Read the model definition and answer for the solid it produces. Units are mm, in the model's axes. Face numbers are marked on the shaded views. A direction names the side the tool comes from. Give positions to 0.01 mm unless a question says otherwise; leave off trailing zeros. Write each loop counter-clockwise with the first axis right and the second up, starting at its lowest first coordinate (ties: lowest second). Pieces come first, ordered by that corner, then holes. Notation, with made-up numbers: (-37.5, -18.5) - (19.5, -18.5) arc R21 cw to (19.5, 6.5) - close; hole circle Ø8 at (-27, -7). An arc over 180 degrees is marked (long way). Use CSV: the item, a comma, the result in double quotes. Start each with the question number.
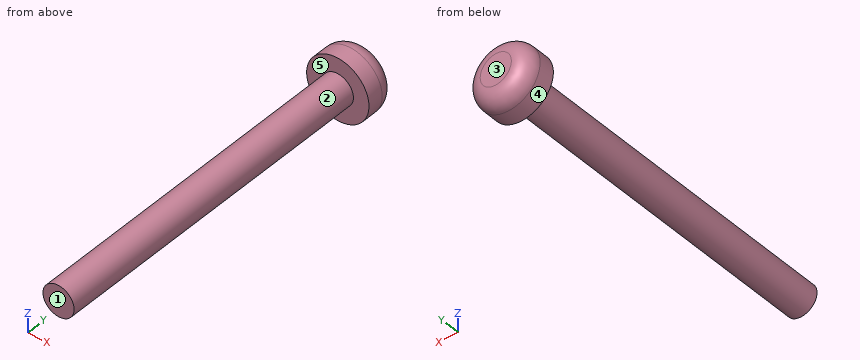
from build123d import *

# Parameters (mm, degrees)
SKETCH1_R           = 3
BOSS_EXTRUDE1_DEPTH = 3
FILLET1_R           = 1.5
SKETCH2_R           = 1.5
BOSS_EXTRUDE2_DEPTH = 31.75


with BuildPart() as part:
    # Sketch1 → Boss-Extrude1 (new body)
    with BuildSketch(Plane(origin=(0, 0, 0), x_dir=(1, 0, 0), z_dir=(0, 1, 0))):
        Circle(SKETCH1_R)
    extrude(amount=BOSS_EXTRUDE1_DEPTH)

    # Fillet1
    fillet1_edges = [part.edges().sort_by_distance(p)[0] for p in [
        (-3, 3, 0),
    ]]
    fillet(fillet1_edges, radius=FILLET1_R)

    # Sketch2 → Boss-Extrude2 (add)
    with BuildSketch(Plane.XZ):
        Circle(SKETCH2_R)
    extrude(amount=BOSS_EXTRUDE2_DEPTH)


solid = part.part
(1) Which of the six approach directions +Z, -Z, +X, -X, +Y, -Y give full straight-line access (tool end or side, diameter ignored) to the marked faces 4 and 5?
(2) The part is cut by section A-A on y = -9. Write down the section's boundary in (x, z), plus the area to 3 significant figures.
(3) For a pull along Y with two mould halves and no side action, classify the marked faces 1, 2 and 3 as pulls with the +Y half, pulls with the -Y half, needs draft (parallel to the pull), parting line crosses it, or undercut.
(4) Consider probe 1 along Z at (x, y) = (-1, -16); probe 2 along Z at (x, y) = (1.25, -9); probe 3 along X at (y, z) = (-14, -0.5). Determine where each line is inside the solid, lowest interval first.
(5) Given P1, Ø3, axis at x = -2, y = -6.5, coming from the -Z side; P2, Ø1, axis at x = -1, z = -2.5, coming from the -Y side; P3, Ø3, axis at x = -2, y = -25.5, coming from the +Z side, each flat-ended and moving along its own axis, determine where each tip first touches the part or whether it passes through.
Reported:
1,face 4,"+Y, -Y"
1,face 5,"-Y"
2,outline,"circle Ø3 at (0, 0)"
2,area,"7.07 mm²"
3,face 1,"pulls with the -Y half"
3,face 2,"needs draft"
3,face 3,"pulls with the +Y half"
4,probe 1,"-1.12 to 1.12"
4,probe 2,"-0.83 to 0.83"
4,probe 3,"-1.41 to 1.41"
5,P1,"z = -1.41"
5,P2,"y = 0"
5,P3,"z = 1.41"
